```python
from build123d import *
from build123d.topology import SkipClean

# Parameters (mm, degrees)
SKETCH1_R           = 93.345
SKETCH1_R_2         = 83.82
BOSS_EXTRUDE1_DEPTH = 6.35
SKETCH2_R           = 88.9
SKETCH2_R_2         = 83.82
BOSS_EXTRUDE2_DEPTH = 19.05
CUT_EXTRUDE1_DEPTH  = 38.1
CIRPATTERN1_COUNT   = 4
SKETCH4_R           = 88.9
SKETCH4_R_2         = 83.82
BOSS_EXTRUDE3_DEPTH = 6.35


with BuildPart() as part:
    # Sketch1 → Boss-Extrude1 (new, symmetric)
    with BuildSketch(Plane(origin=(0, 0, 0), x_dir=(1, 0, 0), z_dir=(0, 1, 0))):
        with Locations(Location((0, 0, 0), (0, 0, 270))):
            Circle(SKETCH1_R)
        with Locations(Location((0, 0, 0), (0, 0, 270))):
            Circle(SKETCH1_R_2, mode=Mode.SUBTRACT)
    extrude(amount=BOSS_EXTRUDE1_DEPTH, both=True)

    # Sketch2 → Boss-Extrude2 (add, symmetric)
    with BuildSketch(Plane(origin=(0, 0, 0), x_dir=(1, 0, 0), z_dir=(0, 1, 0))):
        with Locations(Location((0, 0, 0), (0, 0, 90))):
            Circle(SKETCH2_R)
        with Locations(Location((0, 0, 0), (0, 0, 270))):
            Circle(SKETCH2_R_2, mode=Mode.SUBTRACT)
    extrude(amount=BOSS_EXTRUDE2_DEPTH, both=True)

    # Sketch3 → Cut-Extrude1 (cut, symmetric)
    with BuildSketch(Plane(origin=(0, 0, 0), x_dir=(1, 0, 0), z_dir=(0, 1, 0))):
        with BuildLine():
            Line((0, 0), (-22.96498538, 85.882591056))
            ThreePointArc((-22.96498538, 85.882591056), (0.022788865, 88.899997079), (23.00901311, 85.870805957))
            Line((23.00901311, 85.870805957), (0, 0))
        make_face()
    cut_extrude1 = extrude(amount=CUT_EXTRUDE1_DEPTH, both=True, mode=Mode.SUBTRACT)

    # CirPattern1: Cut-Extrude1 ×4 about axis
    cirpattern1_axis = Axis((0, 19.05, 0), (0, -1, 0))
    for i in range(1, CIRPATTERN1_COUNT):
        add(cut_extrude1.rotate(cirpattern1_axis, i * 360 / CIRPATTERN1_COUNT), mode=Mode.SUBTRACT)

    # Sketch4 → Boss-Extrude3 (add, symmetric)
    with SkipClean():  # the faces are left unmerged after this step: merging them gives an invalid solid
        with BuildSketch(Plane(origin=(0, 0, 0), x_dir=(1, 0, 0), z_dir=(0, 1, 0))):
            Circle(SKETCH4_R)
            with Locations(Location((0, 0, 0), (0, 0, 104.970625291))):
                Circle(SKETCH4_R_2, mode=Mode.SUBTRACT)
        extrude(amount=BOSS_EXTRUDE3_DEPTH, both=True)


solid = part.part
```
Work out the finished part from the listing and answer in its coordinate system (mm). A direction names the side the tool comes from. Give positions to 0.01 mm unless a question says otherwise; leave off trailing zeros. Write each loop counter-clockwise with the first axis right and the second up, starting at its lowest first coordinate (ties: lowest second). Pieces come first, ordered by that corner, then holes. Notation, with made-up numbers: (2.25, -36) - (23.25, -36) arc R12 cw to (23.25, -13) - close; hole circle Ø4 at (-29.5, 1). An arc over 180 degrees is marked (long way). Use one line per item in the form item = value.
1. Each of these flat-tipped pins is pushed along its axis until it touches: pin 1 Ø5 at (y, z) = (6, -52) entering from +X; pin 2 Ø8 at (x, y) = (-40, -3.5) entering from -Z; pin 3 Ø8.5 at (x, z) = (-85.5, -6) entering from -Y. Where does it stop, or does it pass through?
Filled in:
pin_1 = 79.14
pin_2 = -86.12
pin_3 = -6.35
2. A cutting plane is placed at B-B (z = 0). Write down the section's boundary in (x, y) (3 decimals).
Filled in:
outline = (-93.345, -6.35) - (-83.82, -6.35) - (-83.82, 6.35) - (-93.345, 6.35) - close; (83.82, -6.35) - (93.345, -6.35) - (93.345, 6.35) - (83.82, 6.35) - close
3. Determine the mould class of faces 4 (the face through (83.45, -12.61, 22.36)), 5 (the face through (-61, 19.05, 59)), 6 (the face through (22.3, -12.6, 83.4)) for opening direction Z: released by +Z, released by -Z, zero draft, split by the parting line, or undercut.
Filled in:
face_4 = undercut
face_5 = zero draft
face_6 = released by +Z
4. A cutting plane is placed at C-C (x = 0). Write down the section's boundary in (y, z) (3 decimals).
Filled in:
outline = (-6.35, -93.345) - (6.35, -93.345) - (6.35, -83.82) - (-6.35, -83.82) - close; (-6.35, 83.82) - (6.35, 83.82) - (6.35, 93.345) - (-6.35, 93.345) - close
5. A cutting plane is placed at D-D (z = -39.5). Write down the section's boundary in (x, y).
Filled in:
outline = (-84.58, -6.35) - (-79.64, -6.35) - (-79.64, -19.05) - (-73.93, -19.05) - (-73.93, 19.05) - (-79.64, 19.05) - (-79.64, 6.35) - (-84.58, 6.35) - close; (73.93, -19.05) - (79.64, -19.05) - (79.64, -6.35) - (84.58, -6.35) - (84.58, 6.35) - (79.64, 6.35) - (79.64, 19.05) - (73.93, 19.05) - close
6. Consider L1, parallel to X at y = 2.5, z = 0 (3 decimals); L2, parallel to Z at x = 65.5, y = -5.5; L3, parallel to Z at x = -26, y = 3.5. Determine where each line is inside the solid, lowest interval first.
Filled in:
L1 = -93.345 to -83.82, 83.82 to 93.345
L2 = -66.51 to -52.3, 52.3 to 66.51
L3 = -89.65 to -79.69, 79.69 to 89.65
7. A cutting plane is placed at A-A (y = 14). Write down the section's boundary in (x, z), and give its area (3 significant figures).
Filled in:
outline = (-85.88, 22.96) - (-80.98, 21.65) arc R83.82 cw to (-21.69, 80.96) - (-23.01, 85.87) arc R88.9 ccw to start; (-85.87, -23.01) arc R88.9 ccw to (-22.96, -85.88) - (-21.65, -80.98) arc R83.82 cw to (-80.96, -21.69) - close; (21.65, 80.98) arc R83.82 cw to (80.96, 21.69) - (85.87, 23.01) arc R88.9 ccw to (22.96, 85.88) - close; (21.69, -80.96) - (23.01, -85.87) arc R88.9 ccw to (85.88, -22.96) - (80.98, -21.65) arc R83.82 cw to start
area = 1,840 mm^2
8. For faces 1 (the face through (63.34, -12.61, -62.38)), 2 (the face through (-83, 6.35, -14)), 3 (the face through (62.38, -12.61, 63.34)), determine the directions among +Z, -Z, +X, -X, +Y, -Y from which every point of the face is accessible in a straight line to the end or side of a thin tool.
Filled in:
face_1 = -Z, +X, -Y
face_2 = +Y
face_3 = +Z, +X, -Y
